Source: CAD feature listing. Evaluate the final solid. Frame: model axes, mm. Face numbers are marked on the shaded views. A direction names the side the tool comes from. Round coordinates to 2 decimals unless told otherwise and drop trailing zeros. Order: outer loops, then holes, each group sorted by start corner. A loop starts at its lowest first (then second) coordinate and runs counter-clockwise, first axis right, second up. Notation, with made-up numbers: (83.25, -34) -> (104.25, -34) arc R8 cw to (104.25, -29) -> close; hole circle Ø4 at (55, -8.75). An arc over 180 degrees is marked (long way). One line per item, written item: value. Start each with the question number.
1) Section C-C (y = -22). Return the cut outline in (x, z), and give its area (3 significant figures).
2) Reachability of the marked faces 4, 5 and 6 from +Z, -Z, +X, -X, +Y, -Y: full face, straight path, thin tool, end or side. Return the list, or none.
3) Section D-D (z = -7). Return the cut outline in (x, y), and give its area (3 significant figures).
4) Section B-B (z = -16.5). Return the cut outline in (x, y), and give its area (3 significant figures).
5) Ray query, L1, parallel to X at y = -20, z = -4.5; L2, parallel to X at y = -37, z = -3.5; L3, parallel to X at y = -41, z = 0.5. Return the intervals inside material, ascending.
6) Mould query, pull axis X, two halves, no side actions, for the marked faces 1, 2 and 3. Classes: pulls with the +X half, pulls with the -X half, needs draft (parallel to the pull), parting line crosses it, or undercut.
7) Pin query (flat end, axial travel): P1, Ø4, axis at x = -11, z = 17, coming from the -Y side; P2, Ø6, axis at x = 11.5, y = -10.5, coming from the +Z side; P3, Ø8, axis at x = 13, y = -13.5, coming from the -Z side. Return the tip coordinate at first contact, or that it passes through.
8) Section A-A (y = -39). Return the cut outline in (x, z), and give its area (3 significant figures).
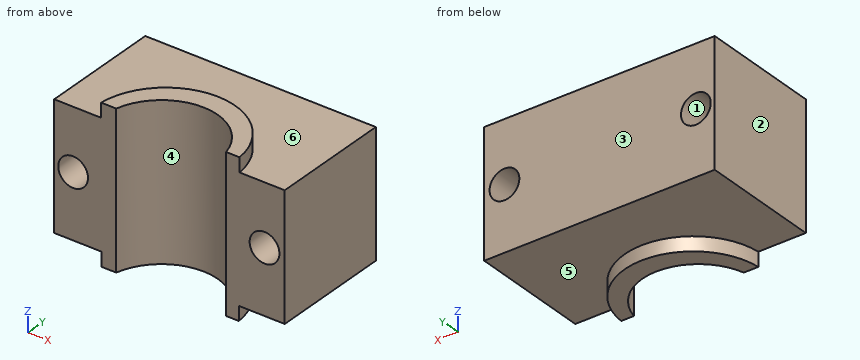
```python
from build123d import *

# Parameters (mm, degrees)
F0_W     = 82.4199393392
F0_H     = 44.8248814791
F0_R     = 5.3237338681
F1_DEPTH = 43.18
F3_DEPTH = 50.8
F5_DEPTH = 5.08
F7_DEPTH = 5.08


with BuildPart() as f1:
    # F0 (on Front) → F1 (new body)
    with BuildSketch(Plane.XZ):
        with Locations((-3.7354081869, -4.2173946276)):
            Rectangle(F0_W, F0_H)
        with Locations((-38.1975471973, -3.7354065571)):
            Circle(F0_R, mode=Mode.SUBTRACT)
        with Locations((30.2447415888, -3.7354065571)):
            Circle(F0_R, mode=Mode.SUBTRACT)
    extrude(amount=F1_DEPTH)

    # F2 (on face) → F3 (cut)
    with BuildSketch(Plane(origin=(0, 0, -26.6298353672), x_dir=(1, 0, 0), z_dir=(0, 0, -1))):
        with BuildLine():
            Line((16.5080875158, 43.18), (-22.7739289403, 43.18))
            ThreePointArc((-22.7739289403, 43.18), (-3.1329207122, 27.6417514992), (16.5080875158, 43.18))
        make_face()
    extrude(amount=-F3_DEPTH, mode=Mode.SUBTRACT)

    # F4 (on face) → F5 (join)
    with BuildSketch(Plane(origin=(0, 0, -26.6298353672), x_dir=(1, 0, 0), z_dir=(0, 0, -1))):
        with BuildLine():
            Line((-22.7739289403, 43.18), (-27.9714372009, 43.18))
            ThreePointArc((-27.9714372009, 43.18), (-3.4506693482, 20.3081134408), (21.0700985044, 43.18))
            Line((21.0700985044, 43.18), (16.5080875158, 43.18))
            ThreePointArc((16.5080875158, 43.18), (-3.1329207122, 27.6417514992), (-22.7739289403, 43.18))
        make_face()
    extrude(amount=F5_DEPTH)

    # F6 (on face) → F7 (join)
    with BuildSketch(Plane.XY.offset(18.1950461119)):
        with BuildLine():
            Line((16.5080875158, -43.18), (21.3290713727, -43.18))
            ThreePointArc((21.3290713727, -43.18), (-3.4313481301, -20.4979947498), (-28.191767633, -43.18))
            Line((-28.191767633, -43.18), (-22.7739289403, -43.18))
            ThreePointArc((-22.7739289403, -43.18), (-3.1329207122, -27.6417514992), (16.5080875158, -43.18))
        make_face()
    extrude(amount=F7_DEPTH)


solid = f1.part
```
Findings:
1. outline: (-44.95, -26.63) -> (-12.41, -26.63) -> (-12.41, -31.71) -> (5.51, -31.71) -> (5.51, -26.63) -> (37.47, -26.63) -> (37.47, 18.2) -> (5.08, 18.2) -> (5.08, 23.28) -> (-11.94, 23.28) -> (-11.94, 18.2) -> (-44.95, 18.2) -> close; hole circle Ø10.65 at (-38.2, -3.74); hole circle Ø10.65 at (30.24, -3.74)
1. area: 3,690 mm2
2. face 4: +Z, -Z, -Y
2. face 5: -Z, +Y
2. face 6: +Z, +Y
3. outline: (-44.95, -43.18) -> (-42.4, -43.18) -> (-42.4, 0) -> (-44.95, 0) -> close; (-33.99, -43.18) -> (-22.77, -43.18) arc R20.18 cw to (16.51, -43.18) -> (26.04, -43.18) -> (26.04, 0) -> (-33.99, 0) -> close; (34.45, -43.18) -> (37.47, -43.18) -> (37.47, 0) -> (34.45, 0) -> close
3. area: 2,380 mm2
4. outline: (-44.95, -43.18) -> (-22.77, -43.18) arc R20.18 cw to (16.51, -43.18) -> (37.47, -43.18) -> (37.47, 0) -> (-44.95, 0) -> close
4. area: 3,100 mm2
5. L1: -44.95 to -43.47, -32.93 to 24.98, 35.51 to 37.47
5. L2: -44.95 to -43.52, -32.88 to -20.17, 13.9 to 24.93, 35.56 to 37.47
5. L3: -44.95 to -41.42, -34.97 to -22.13, 15.86 to 27.02, 33.47 to 37.47
6. face 1: undercut
6. face 2: pulls with the -X half
6. face 3: needs draft
7. P1: y = -30.22
7. P2: z = 18.2
7. P3: z = -26.63
8. outline: (-44.95, -26.63) -> (-27.32, -26.63) -> (-27.32, -31.71) -> (-21.28, -31.71) -> (-21.28, 23.28) -> (-27.46, 23.28) -> (-27.46, 18.2) -> (-44.95, 18.2) -> close; (15.02, -31.71) -> (20.41, -31.71) -> (20.41, -26.63) -> (37.47, -26.63) -> (37.47, 18.2) -> (20.6, 18.2) -> (20.6, 23.28) -> (15.02, 23.28) -> close; hole circle Ø10.65 at (-38.2, -3.74); hole circle Ø10.65 at (30.24, -3.74)
8. area: 2,010 mm2
